from build123d import *

# Parameters (mm, degrees)
CUT_EXTRUDE2_DEPTH      = 7
CUT_EXTRUDE2_DEPTH_BACK = 7


with BuildPart() as part:
    # Sketch1 → Revolve1 (revolve)
    with BuildSketch(Plane.XY):
        with BuildLine():
            Line((-6, 0), (6, 0))
            ThreePointArc((6, 0), (0, 6), (-6, 0))
        make_face()
    revolve(axis=Axis((-13.60120179, 0, 0), (1, 0, 0)))

    # Sketch2 → Cut-Extrude2 (cut, two sides)
    with BuildSketch(Plane.XY) as cut_extrude2_sk:
        with BuildLine():
            Line((-4.72, 3.704267809), (-4.72, -3.704267809))
            ThreePointArc((-4.72, -3.704267809), (-6, 0), (-4.72, 3.704267809))
        make_face()
        with BuildLine():
            Line((4.72, 3.704267809), (4.72, -3.704267809))
            ThreePointArc((4.72, -3.704267809), (6, 0), (4.72, 3.704267809))
        make_face()
    extrude(amount=CUT_EXTRUDE2_DEPTH, mode=Mode.SUBTRACT)
    extrude(cut_extrude2_sk.sketch, amount=-CUT_EXTRUDE2_DEPTH_BACK, mode=Mode.SUBTRACT)

    # Sketch3 → Cut-Revolve1 (revolve, cut)
    with BuildSketch(Plane.XY, mode=Mode.PRIVATE) as cut_revolve1_sk:
        Polygon((-4.72, 3.44), (-3.28, 2), (4.72, 2), (4.72, 0), (-4.72, 0), align=None)
    revolve(cut_revolve1_sk.sketch.rotate(Axis((-7.010525763, 0, 0), (1, 0, 0)), 90), axis=Axis((-7.010525763, 0, 0), (1, 0, 0)), mode=Mode.SUBTRACT)  # turned: the seam where the file's is


solid = part.part
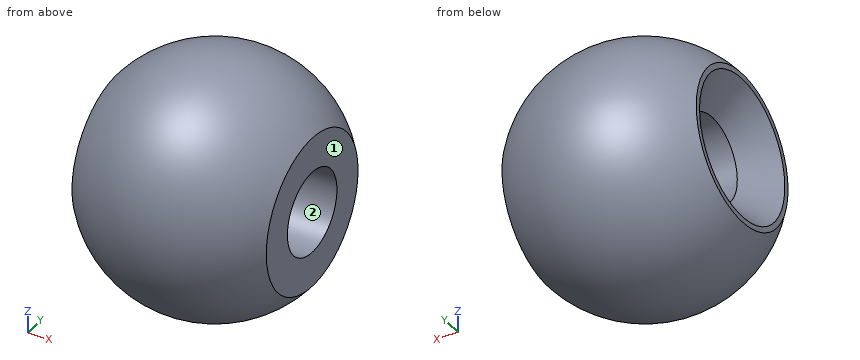
Check sheet for the modelled part. Datum: model origin and axes. Units: mm. Face numbers are marked on the shaded views. Coordinates: 2 decimals unless noted, no trailing zeros. Write each loop counter-clockwise with the first axis right and the second up, starting at its lowest first coordinate (ties: lowest second). Pieces come first, ordered by that corner, then holes.
Item 1: Scan lines: probe 1 along Y at (x, z) = (1, 0); probe 2 along Z at (x, y) = (-0.25, -1.5); probe 3 along Z at (x, y) = (3, -0.25). Record each from-to range of solid material in increasing order.
Numbers:
probe 1: y = -5.92 to -2, 2 to 5.92
probe 2: z = -5.8 to -1.32, 1.32 to 5.8
probe 3: z = -5.19 to -1.98, 1.98 to 5.19
Item 2: Cross-section at D-D on z = 4.75. Record the boundary of the cut face in (x, y).
Numbers:
outline: circle Ø7.33 at (0, 0)
Item 3: Depth check by flat-ended pin: pin 1 Ø1.5 at (x, z) = (2.5, -2) entering from +Y; pin 2 Ø2.5 at (y, z) = (0, 0) entering from -X; pin 3 Ø4 at (x, y) = (3, -4) entering from +Z; pin 4 Ø1 at (y, z) = (4.5, -3) entering from +X. Enter the tip coordinate at first touch or a pass-through.
Numbers:
pin 1: stops at y = 5.48
pin 2: passes through
pin 3: stops at z = 5.2
pin 4: stops at x = 3.45
Item 4: Cross-section at B-B on x = -1.5. Record the boundary of the cut face in (y, z).
Numbers:
outline: circle Ø11.62 at (0, 0); hole circle Ø4 at (0, 0)
Item 5: Cross-section at A-A on z = 0. Record the boundary of the cut face in (x, y).
Numbers:
outline: (-4.72, -3.7) arc R6 ccw to (4.72, -3.7) - (4.72, -2) - (-3.28, -2) - (-4.72, -3.44) - close; (-4.72, 3.44) - (-3.28, 2) - (4.72, 2) - (4.72, 3.7) arc R6 ccw to (-4.72, 3.7) - close
Item 6: Mould release check, pull along Y, two halves, no side actions. Record for the marked faces 1 and 2: released by +Y, released by -Y, zero draft, split by the parting line, or undercut.
Numbers:
face 1: zero draft
face 2: undercut
Item 7: Cross-section at C-C on y = -5. Record the boundary of the cut face in (x, z).
Numbers:
outline: circle Ø6.63 at (0, 0)
